Geometry check sheet. Reference: the model listing, model coordinates, mm. A direction names the side the tool comes from. Give positions to 0.01 mm unless a question says otherwise; leave off trailing zeros. Loops run counter-clockwise (first coordinate to the right, second up) from the corner with the lowest first, then second, coordinate; pieces in that order, holes last. Notation, with made-up numbers: (-26, 75.5) -> (24, 75.5) arc R9 cw to (24, 88.5) -> close; hole circle Ø1 at (41, 40.5). An arc over 180 degrees is marked (long way). Answer as a JSON object with one key per item and string values.
from build123d import *

# Parameters (mm, degrees)
F0_W          = 60
F0_H          = 180
F0_R          = 12.75
F0_R_2        = 2.5
F1_DEPTH      = 3
F2_R          = 18
F2_R_2        = 12.75
F3_DEPTH      = 2.6
F4_W          = 60
F4_H          = 70
F4_W_2        = 54
F4_H_2        = 64
F5_DEPTH      = 40
F6_W          = 5
F6_H          = 5
F6_W_2        = 10
F6_H_2        = 3
F6_W_3        = 3
F6_H_3        = 10
F7_DEPTH      = 37
F8_R          = 1.6
F9_DEPTH      = 28
F10_W         = 3
F10_H         = 70
F11_DEPTH     = 70
F13_R         = 20.5
F14_DEPTH     = 3
F16_DEPTH     = 5
F17_R         = 3.075
F18_DEPTH     = 6
F19_R         = 3.1
F20_DEPTH     = 6
F22_DEPTH     = 5
F23_R         = 5
F24_T1_DEPTH  = 47.5
F24_T3_DEPTH  = 50.5
F24_T5_DEPTH  = 15.5
F24_S9_W      = 5.1
F24_S9_H      = 5.1
F24_T10_DEPTH = 5.1
F24_S15_W     = 5.1
F24_S15_H     = 5.1
F24_T16_DEPTH = 5.1
F24_S21_W     = 5.1
F24_S21_H     = 5.1
F24_T22_DEPTH = 5.1
F24_S27_W     = 5.1
F24_S27_H     = 5.1
F24_T28_DEPTH = 5.1
F24_S33_W     = 5.1
F24_S33_H     = 5.1
F24_T34_DEPTH = 5.1
F24_T40_DEPTH = 60
F24_T46_DEPTH = 60
F24_T52_DEPTH = 60
F24_T58_DEPTH = 60


# Not quite as in the source:
# - a fillet or chamfer that OpenCascade refuses, or shapes differently, is made with other operations: its cross-section is extruded or revolved along the edge and cut away or added


with BuildPart() as f1:
    # F0 (on Front) → F1 (new body)
    with BuildSketch(Plane.XZ):
        Rectangle(F0_W, F0_H)
        with Locations((0, -55)):
            Circle(F0_R, mode=Mode.SUBTRACT)
        with Locations((-17.5, 30)):
            Circle(F0_R_2, mode=Mode.SUBTRACT)
        with Locations((-17.5, 75)):
            Circle(F0_R_2, mode=Mode.SUBTRACT)
        with Locations((17.5, 30)):
            Circle(F0_R_2, mode=Mode.SUBTRACT)
        with Locations((17.5, 75)):
            Circle(F0_R_2, mode=Mode.SUBTRACT)
    extrude(amount=-F1_DEPTH)

    # F2 (on face) → F3 (join)
    with BuildSketch(Plane.XZ):
        with Locations((0, -55)):
            Circle(F2_R)
        with Locations((0, -55)):
            Circle(F2_R_2, mode=Mode.SUBTRACT)
    extrude(amount=F3_DEPTH)

    # F4 (on face) → F5 (join)
    with BuildSketch(Plane.XZ):
        with Locations((0, -55)):
            Rectangle(F4_W, F4_H)
        with Locations((0, -55)):
            Rectangle(F4_W_2, F4_H_2, mode=Mode.SUBTRACT)
    extrude(amount=F5_DEPTH)

    # F6 (on face) → F7 (join)
    with BuildSketch(Plane.XZ):
        with Locations((-24.5, -25.5)):
            Rectangle(F6_W, F6_H)
        with Locations((0, -24.5)):
            Rectangle(F6_W_2, F6_H_2)
        with Locations((24.5, -25.5)):
            Rectangle(F6_W, F6_H)
        with Locations((25.5, -55)):
            Rectangle(F6_W_3, F6_H_3)
        with Locations((-25.5, -55)):
            Rectangle(F6_W_3, F6_H_3)
        with Locations((24.5, -84.5)):
            Rectangle(F6_W, F6_H)
        with Locations((0, -85.5)):
            Rectangle(F6_W_2, F6_H_2)
        with Locations((-24.5, -84.5)):
            Rectangle(F6_W, F6_H)
    extrude(amount=F7_DEPTH)

    # F8 (on face) → F9 (cut)
    with BuildSketch(Plane.XZ.offset(37)):
        with Locations((24.5, -25.5)):
            Circle(F8_R)
        with Locations((-24.5, -25.5)):
            Circle(F8_R)
        with Locations((24.5, -84.5)):
            Circle(F8_R)
        with Locations((-24.5, -84.5)):
            Circle(F8_R)
    extrude(amount=-F9_DEPTH, mode=Mode.SUBTRACT)

    # F10 (on face) → F11 (join)
    with BuildSketch(Plane.YZ.offset(30)):
        with Locations((1.5, -55)):
            Rectangle(F10_W, F10_H)
    extrude(amount=F11_DEPTH)

    # F13 (on face) → F14 (cut, through all)
    with BuildSketch(Plane.XZ):
        with Locations((65, -55)):
            Circle(F13_R)
    extrude(amount=-F14_DEPTH, mode=Mode.SUBTRACT)

    # F15 (on face) → F16 (join)
    with BuildSketch(Plane.XZ):
        Polygon((100, -20), (30, -20), (30, -23), (97, -23), (97, -87), (30, -87), (30, -90), (100, -90), (100, -87), (100, -23), align=None)
    extrude(amount=F16_DEPTH)

    # F17 (on face) → F18 (cut, through all)
    with BuildSketch(Plane.YZ.offset(30)):
        with Locations((-22.5, -55)):
            Circle(F17_R)
    extrude(amount=-F18_DEPTH, mode=Mode.SUBTRACT)

    # F19 (on face) → F20 (cut, through all)
    with BuildSketch(Plane.XY.offset(-20)):
        with Locations((0, -20)):
            Circle(F19_R)
    extrude(amount=-F20_DEPTH, mode=Mode.SUBTRACT)

    # F21 (on face) → F22 (join)
    with BuildSketch(Plane.XZ):
        Polygon((30, -20), (30, 90), (27, 90), (21.6846410185, 90), (-27, 90), (-30, 90), (-30, -20), (-27, -20), (-27, 87), (27, 87), (27, -20), align=None)
    extrude(amount=F22_DEPTH)

    # F23
    f23_edges = [f1.edges().sort_by_distance(p)[0] for p in [
        (35, 3, -90),
        (-30, 3, 0),
        (0, 3, 90),
        (30, 3, 35),
        (65, 3, -20),
        (100, 3, -55),
    ]]
    fillet(f23_edges, radius=F23_R)

    # F24: fillet of radius 5 on 8 edges, made by hand

    # F24_s2 → F24_t1 (cut)
    with BuildSketch(Plane.XZ.offset(5)):
        with BuildLine():
            ThreePointArc((30, -25), (28.5355339059, -21.4644660941), (25, -20))
            Line((25, -20), (30, -20))
            Line((30, -20), (30, -25))
        make_face()
        with BuildLine():
            ThreePointArc((-30, -25), (-28.5355339059, -21.4644660941), (-25, -20))
            Line((-25, -20), (-30, -20))
            Line((-30, -20), (-30, -25))
        make_face()
        with BuildLine():
            ThreePointArc((25, -90), (28.5355339059, -88.5355339059), (30, -85))
            Line((30, -85), (30, -90))
            Line((30, -90), (25, -90))
        make_face()
    extrude(amount=F24_T1_DEPTH, mode=Mode.SUBTRACT)

    # F24_s4 → F24_t3 (cut)
    with BuildSketch(Plane.XZ.offset(2)):
        with BuildLine():
            ThreePointArc((-25, -90), (-28.5355339059, -88.5355339059), (-30, -85))
            Line((-30, -85), (-30, -90))
            Line((-30, -90), (-25, -90))
        make_face()
    extrude(amount=F24_T3_DEPTH, mode=Mode.SUBTRACT)

    # F24_s6 → F24_t5 (cut)
    with BuildSketch(Plane.XZ.offset(2)):
        with BuildLine():
            ThreePointArc((100, -25), (98.5355339059, -21.4644660941), (95, -20))
            Line((95, -20), (100, -20))
            Line((100, -20), (100, -25))
        make_face()
        with BuildLine():
            ThreePointArc((95, -90), (98.5355339059, -88.5355339059), (100, -85))
            Line((100, -85), (100, -90))
            Line((100, -90), (95, -90))
        make_face()
        with BuildLine():
            ThreePointArc((25, 90), (28.5355339059, 88.5355339059), (30, 85))
            Line((30, 85), (30, 90))
            Line((30, 90), (25, 90))
        make_face()
        with BuildLine():
            ThreePointArc((-30, 85), (-28.5355339059, 88.5355339059), (-25, 90))
            Line((-25, 90), (-30, 90))
            Line((-30, 90), (-30, 85))
        make_face()
    extrude(amount=F24_T5_DEPTH, mode=Mode.SUBTRACT)


with BuildPart() as f24_tool8:
    # F24_s9 → F24_t10 (new body)
    with BuildSketch(Plane.YZ.offset(-25)):
        with Locations((0.55, 87.55)):
            Rectangle(F24_S9_W, F24_S9_H)
    extrude(amount=-F24_T10_DEPTH)

    # F24_s11 → F24_t12 (revolve, cut)
    with BuildSketch(Plane(origin=(-25, -2, 85), x_dir=(0, -0.7071067812, -0.7071067812), z_dir=(0, 0.7071067812, -0.7071067812))):
        with BuildLine():
            ThreePointArc((0, -5), (5, 0), (0, 5))
            Line((0, 5), (0, -5))
        make_face()
    revolve(axis=Axis((-25, -2, 85), (-1, 0, 0)), mode=Mode.SUBTRACT)


with BuildPart() as f1_1:
    add(f1.part)

    # F24_t7: cut F24_tool8
    add(f24_tool8.part, mode=Mode.SUBTRACT)


with BuildPart() as f24_tool14:
    # F24_s15 → F24_t16 (new body)
    with BuildSketch(Plane.XY.offset(85)):
        with Locations((27.55, 0.55)):
            Rectangle(F24_S15_W, F24_S15_H)
    extrude(amount=F24_T16_DEPTH)

    # F24_s17 → F24_t18 (revolve, cut)
    with BuildSketch(Plane(origin=(25, -2, 85), x_dir=(-0.7071067812, -0.7071067812, 0), z_dir=(-0.7071067812, 0.7071067812, 0))):
        with BuildLine():
            ThreePointArc((0, -5), (5, 0), (0, 5))
            Line((0, 5), (0, -5))
        make_face()
    revolve(axis=Axis((25, -2, 85), (0, 0, 1)), mode=Mode.SUBTRACT)


with BuildPart() as f1_2:
    add(f1_1.part)

    # F24_t13: cut F24_tool14
    add(f24_tool14.part, mode=Mode.SUBTRACT)


with BuildPart() as f24_tool20:
    # F24_s21 → F24_t22 (new body)
    with BuildSketch(Plane.XY.offset(-85)):
        with Locations((97.55, 0.55)):
            Rectangle(F24_S21_W, F24_S21_H)
    extrude(amount=-F24_T22_DEPTH)

    # F24_s23 → F24_t24 (revolve, cut)
    with BuildSketch(Plane(origin=(95, -2, -85), x_dir=(-0.7071067812, -0.7071067812, 0), z_dir=(0.7071067812, -0.7071067812, 0))):
        with BuildLine():
            ThreePointArc((0, -5), (5, 0), (0, 5))
            Line((0, 5), (0, -5))
        make_face()
    revolve(axis=Axis((95, -2, -85), (0, 0, -1)), mode=Mode.SUBTRACT)


with BuildPart() as f1_3:
    add(f1_2.part)

    # F24_t19: cut F24_tool20
    add(f24_tool20.part, mode=Mode.SUBTRACT)


with BuildPart() as f24_tool26:
    # F24_s27 → F24_t28 (new body)
    with BuildSketch(Plane.YZ.offset(95)):
        with Locations((0.55, -22.45)):
            Rectangle(F24_S27_W, F24_S27_H)
    extrude(amount=F24_T28_DEPTH)

    # F24_s29 → F24_t30 (revolve, cut)
    with BuildSketch(Plane(origin=(95, -2, -25), x_dir=(0, -0.7071067812, -0.7071067812), z_dir=(0, -0.7071067812, 0.7071067812))):
        with BuildLine():
            ThreePointArc((0, -5), (5, 0), (0, 5))
            Line((0, 5), (0, -5))
        make_face()
    revolve(axis=Axis((95, -2, -25), (1, 0, 0)), mode=Mode.SUBTRACT)


with BuildPart() as f1_4:
    add(f1_3.part)

    # F24_t25: cut F24_tool26
    add(f24_tool26.part, mode=Mode.SUBTRACT)


with BuildPart() as f24_tool32:
    # F24_s33 → F24_t34 (new body)
    with BuildSketch(Plane.XY.offset(-85)):
        with Locations((-27.55, 0.55)):
            Rectangle(F24_S33_W, F24_S33_H)
    extrude(amount=-F24_T34_DEPTH)

    # F24_s35 → F24_t36 (revolve, cut)
    with BuildSketch(Plane(origin=(-25, -2, -85), x_dir=(0.7071067812, -0.7071067812, 0), z_dir=(0.7071067812, 0.7071067812, 0))):
        with BuildLine():
            ThreePointArc((0, -5), (5, 0), (0, 5))
            Line((0, 5), (0, -5))
        make_face()
    revolve(axis=Axis((-25, -2, -85), (0, 0, -1)), mode=Mode.SUBTRACT)


with BuildPart() as f1_5:
    add(f1_4.part)

    # F24_t31: cut F24_tool32
    add(f24_tool32.part, mode=Mode.SUBTRACT)


with BuildPart() as f24_tool38:
    # F24_s39 → F24_t40 (new body)
    with BuildSketch(Plane.XZ.offset(-7.5)):
        with BuildLine():
            ThreePointArc((30, -25), (28.5355339059, -21.4644660941), (25, -20))
            Line((25, -20), (30, -20))
            Line((30, -20), (30, -25))
        make_face()
    extrude(amount=F24_T40_DEPTH)

    split(bisect_by=Plane.XY.offset(-23), keep=Keep.BOTTOM)

    split(bisect_by=Plane.XZ, keep=Keep.TOP)


with BuildPart() as f1_6:
    add(f1_5.part)

    # F24_t37: cut F24_tool38
    add(f24_tool38.part, mode=Mode.SUBTRACT)


with BuildPart() as f24_tool44:
    # F24_s45 → F24_t46 (new body)
    with BuildSketch(Plane.XZ.offset(-7.5)):
        with BuildLine():
            ThreePointArc((30, -25), (28.5355339059, -21.4644660941), (25, -20))
            Line((25, -20), (30, -20))
            Line((30, -20), (30, -25))
        make_face()
    extrude(amount=F24_T46_DEPTH)

    split(bisect_by=Plane.XZ, keep=Keep.TOP)

    split(bisect_by=Plane.YZ.offset(27), keep=Keep.BOTTOM)


with BuildPart() as f1_7:
    add(f1_6.part)

    # F24_t43: cut F24_tool44
    add(f24_tool44.part, mode=Mode.SUBTRACT)


with BuildPart() as f24_tool50:
    # F24_s51 → F24_t52 (new body)
    with BuildSketch(Plane.XZ.offset(-7.5)):
        with BuildLine():
            ThreePointArc((-30, -25), (-28.5355339059, -21.4644660941), (-25, -20))
            Line((-25, -20), (-30, -20))
            Line((-30, -20), (-30, -25))
        make_face()
    extrude(amount=F24_T52_DEPTH)

    split(bisect_by=Plane.XZ, keep=Keep.TOP)

    split(bisect_by=Plane.YZ.offset(-27), keep=Keep.TOP)


with BuildPart() as f1_8:
    add(f1_7.part)

    # F24_t49: cut F24_tool50
    add(f24_tool50.part, mode=Mode.SUBTRACT)


with BuildPart() as f24_tool56:
    # F24_s57 → F24_t58 (new body)
    with BuildSketch(Plane.XZ.offset(-7.5)):
        with BuildLine():
            ThreePointArc((25, -90), (28.5355339059, -88.5355339059), (30, -85))
            Line((30, -85), (30, -90))
            Line((30, -90), (25, -90))
        make_face()
    extrude(amount=F24_T58_DEPTH)

    split(bisect_by=Plane.XY.offset(-87), keep=Keep.TOP)

    split(bisect_by=Plane.XZ, keep=Keep.TOP)


with BuildPart() as f1_9:
    add(f1_8.part)

    # F24_t55: cut F24_tool56
    add(f24_tool56.part, mode=Mode.SUBTRACT)


solid = f1_9.part
1) Tool access check on faces 5 (the face through (28, -3, 89)), 6 (the face through (-25, -18, -28)), 7 (the face through (60, 2, -22)). Record the directions out of +Z, -Z, +X, -X, +Y, -Y that give a thin tool (end or side, any length) a straight path to the whole face; none if there is none.
Geometry check:
{"face 5": "+Z, +X, +Y, -Y", "face 6": "-Y", "face 7": "+Z, +X, +Y"}
2) Section check D-D on z = -31. Record the cut outline in (x, y), plus the area to 3 significant figures.
Geometry check:
{"outline": "(-30, -40) -> (-27, -40) -> (-27, 0) -> (27, 0) -> (27, -40) -> (30, -40) -> (30, 0) -> (97, 0) -> (97, -5) -> (100, -5) -> (100, -2) arc R5 ccw to (95, 3) -> (-25, 3) arc R5 ccw to (-30, -2) -> close", "area": "634 mm2"}
3) Draft check along Z on faces 1 (the face through (0, 2, 88)), 2 (the face through (24, -18, -82)), 3 (the face through (48.73, 1.48, -67.47)), 4 (the face through (98, -3, -89)). Enter one of: pulls with the +Z half, pulls with the -Z half, needs draft (parallel to the pull), parting line crosses it, or undercut.
Geometry check:
{"face 1": "pulls with the +Z half", "face 2": "undercut", "face 3": "undercut", "face 4": "pulls with the -Z half"}
4) Material ranges on line 1 along X through (y, z) = (-22.5, -84.5); line 2 along Z through (x, y) = (25.8, -22.5) (3 decimals); line 3 along Y through (x, z) = (0, -23.95), recorded low to high. Write a range as from..to.
Geometry check:
{"line 1": "x = -30..-26.1, -22.9..-22, -5..5, 22..22.9, 26.1..30", "line 2": "z = -89.936..-85.433, -83.567..-82, -60..-58.075, -51.925..-50, -28..-26.433, -24.567..-20.064", "line 3": "y = -37..-23.1, -16.9..3"}
5) Section check B-B on x = 10.5. Record the cut outline in (y, z), plus the area to 3 significant figures.
Geometry check:
{"outline": "(-40, -90) -> (-2, -90) arc R5 ccw to (3, -85) -> (3, -62.23) -> (-2.6, -62.23) -> (-2.6, -69.62) -> (0, -69.62) -> (0, -87) -> (-40, -87) -> close; (-40, -23) -> (0, -23) -> (0, -40.38) -> (-2.6, -40.38) -> (-2.6, -47.77) -> (3, -47.77) -> (3, 85) arc R5 ccw to (-2, 90) -> (-5, 90) -> (-5, 87) -> (0, 87) -> (0, -20) -> (-40, -20) -> close", "area": "779 mm2"}
6) Section check A-A on z = 75. Record the cut outline in (x, y).
Geometry check:
{"outline": "(-30, -5) -> (-27, -5) -> (-27, 0) -> (-20, 0) -> (-20, 3) -> (-25, 3) arc R5 ccw to (-30, -2) -> close; (-15, 0) -> (15, 0) -> (15, 3) -> (-15, 3) -> close; (20, 0) -> (27, 0) -> (27, -5) -> (30, -5) -> (30, -2) arc R5 ccw to (25, 3) -> (20, 3) -> close"}
7) Section check C-C on y = -11.5. Count the separate pieces of the cut face and the enclosed holes in it, plus the area to 3 significant figures.
Geometry check:
{"separate pieces": "1", "enclosed holes": "5", "area": "910 mm2"}
8) Depth check by flat-ended pin: P1, Ø3.5, axis at x = 26, y = -24, coming from the +Z side; P2, Ø2.5, axis at x = -25, z = -85.5, coming from the -Y side; P3, Ø1, axis at x = -25, z = -25, coming from the -Y side. Enter the tip coordinate at first touch or a pass-through.
Geometry check:
{"P1": "stops at z = -20", "P2": "stops at y = -37", "P3": "stops at y = -9"}
